Job drawing, mm, ordinate dimensions from the low corner. One solid piece. A direction names the side the tool comes from. Give positions to 0.01 mm unless a question says otherwise; leave off trailing zeros. Order: outer loops, then holes, each group sorted by start corner. A loop starts at its lowest first (then second) coordinate and runs counter-clockwise, first axis right, second up.
1. Probe line 1 (X direction, y = 10.25, z = 18.5); line 2 (Y direction, x = 11, z = 65); line 3 (X direction, y = 6.5, z = 18). List the from-to ranges inside material, lowest first.
2. Slice it at B-B on z = 50. List the corners of the cut face in (x, y), and give its area (3 significant figures).
3. Which spindle directions (+Z, -Z, +X, -X, +Y, -Y) get a long thin tool onto all of the face, cutting with end or side? Do the marked faces 1 and 2. Say none if no direction does.
4. Drop flat-ended pins along their axis: pin 1 Ø3.5 at (x, y) = (35, 10) entering from +Z; pin 2 Ø7 at (x, y) = (65, 10) entering from +Z; pin 3 Ø7 at (y, z) = (10, 35) entering from +X. Give the stop position or say it passes through.
5. Slice it at C-C on y = 2.5. List the corners of the cut face in (x, z).
6. Slice it at D-D on x = 11. List the corners of the cut face in (y, z).
7. Slice it at A-A on x = 50. List the corners of the cut face in (y, z), and give its area (3 significant figures).
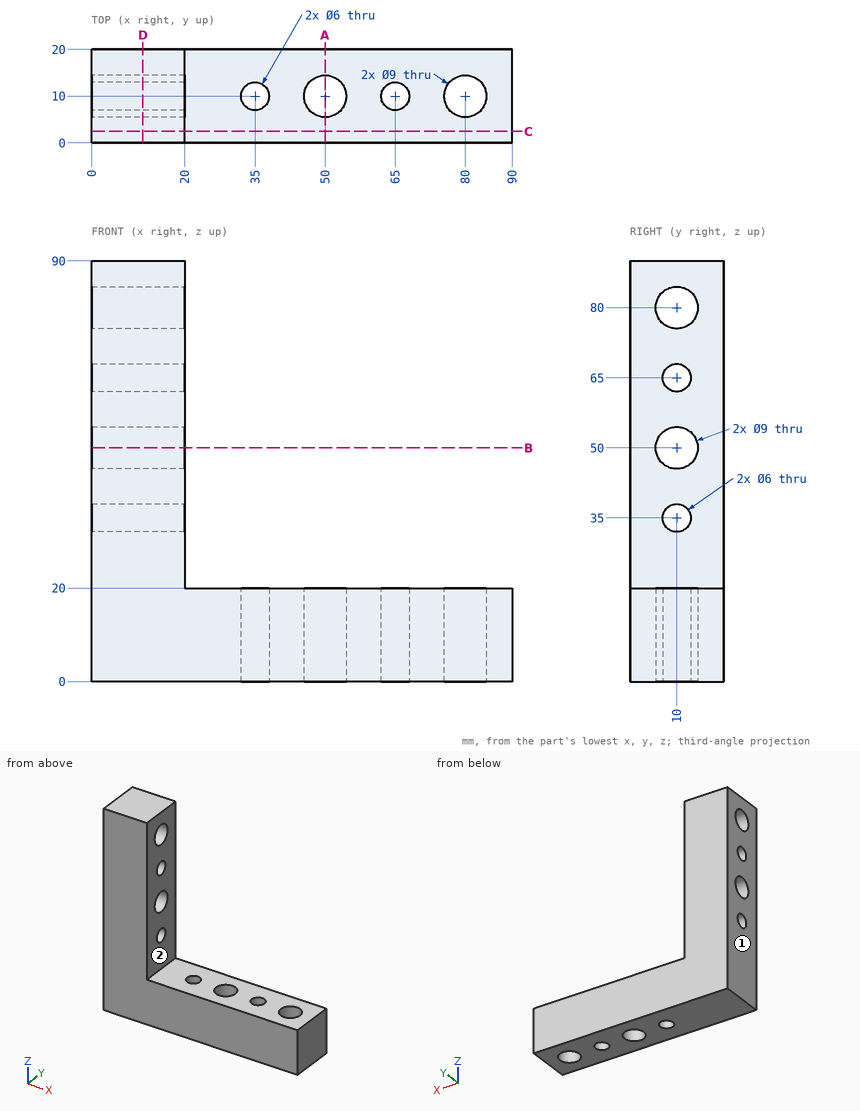
Data:
1. line 1: x = 0 to 32.01, 37.99 to 45.51, 54.49 to 62.01, 67.99 to 75.51, 84.49 to 90
1. line 2: y = 0 to 7, 13 to 20
1. line 3: x = 0 to 47.17, 52.83 to 77.17, 82.83 to 90
2. outline: (0, 0) - (20, 0) - (20, 5.5) - (0, 5.5) - close; (0, 14.5) - (20, 14.5) - (20, 20) - (0, 20) - close
2. area: 220 mm2
3. face 1: +Z, -Z, -X, +Y, -Y
3. face 2: +Z, +X, +Y, -Y
4. pin 1: passes through
4. pin 2: stops at z = 20
4. pin 3: stops at x = 20
5. outline: (0, 0) - (90, 0) - (90, 20) - (20, 20) - (20, 90) - (0, 90) - close
6. outline: (0, 0) - (20, 0) - (20, 90) - (0, 90) - close; hole circle Ø9 at (10, 50); hole circle Ø9 at (10, 80); hole circle Ø6 at (10, 35); hole circle Ø6 at (10, 65)
7. outline: (0, 0) - (5.5, 0) - (5.5, 20) - (0, 20) - close; (14.5, 0) - (20, 0) - (20, 20) - (14.5, 20) - close
7. area: 220 mm2
